Check sheet for the modelled part. Datum: model origin and axes. Units: mm. A direction names the side the tool comes from. Coordinates: 2 decimals unless noted, no trailing zeros. Loops run counter-clockwise (first coordinate to the right, second up) from the corner with the lowest first, then second, coordinate; pieces in that order, holes last.
from build123d import *

# Parameters (mm, degrees)
EXTRUDE_1_DEPTH     = 10
SKETCH_2_R          = 2
CUT_EXTRUDE_1_DEPTH = 13.051970793


with BuildPart() as part:
    # 草图1 → 凸台-拉伸1 (new body)
    with BuildSketch(Plane(origin=(0, 0, 0), x_dir=(1, 0, 0), z_dir=(0, 1, 0))):
        Polygon((-3.5, 0), (3.5, 0), (5, 1.5), (5, 3), (3, 3), (3, 4.5), (-3, 4.5), (-3, 3), (-5, 3), (-5, 1.5), align=None)
    extrude(amount=EXTRUDE_1_DEPTH)

    # 草图2 → 切除-拉伸1 (cut, through all)
    with BuildSketch(Plane.XY):
        with Locations((0, 5)):
            Circle(SKETCH_2_R)
    extrude(amount=-CUT_EXTRUDE_1_DEPTH, mode=Mode.SUBTRACT)


solid = part.part
(1) Section check A-A, the plane x = 0. Enter the section's corners in (y, z).
(2) Section check C-C, the plane y = 0.5. Enter the section's corners in (x, z), plus the area to 4 significant figures.
(3) Set-up check for faces 1 (the face through (3, 5, -4)), 2 (the face through (-5, 5, -2)), 3 (the face through (-3, 5, -4)): record each of +Z, -Z, +X, -X, +Y, -Y from which the full face is reachable in a straight line by a thin tool's end or side.
(4) Scan lines: line 1 along Y through (x, z) = (0, -0.2); line 2 along X through (y, z) = (0.5, -4); line 3 along X through (y, z) = (4.5, -2.95). Record each from-to range of solid material in increasing order.
(5) Section check D-D, the plane y = 5. Enter the section's corners in (x, z).
(6) Gauge pin test, flat ends, axial feed: P1, Ø1, axis at x = 4, y = 6, coming from the -Z side; P2, Ø2.5, axis at x = 0, y = 5, coming from the -Z side; P3, Ø1.6, axis at y = 6, z = -4, coming from the -X side; P4, Ø0.8, axis at y = 3, z = -3.5, coming from the +X side. Record the tip position at first contact, or that the pin passes through.
(7) Section check B-B, the plane z = -0.6. Enter the section's corners in (x, y).
(8) Draft check along Y on faces 4 (the face through (4.2, 4.9, -0.7)), 5 (the face through (0, 0, -2)), 6 (the face through (0, 7, -2)). Enter one of: pulls with the +Y half, pulls with the -Y half, needs draft (parallel to the pull), parting line crosses it, or undercut.
Determined:
1. outline: (0, -4.5) - (3, -4.5) - (3, 0) - (0, 0) - close; (7, -4.5) - (10, -4.5) - (10, 0) - (7, 0) - close
2. outline: (-5, -3) - (-3, -3) - (-3, -4.5) - (3, -4.5) - (3, -3) - (5, -3) - (5, -1.5) - (3.5, 0) - (-3.5, 0) - (-5, -1.5) - close
2. area: 36.75 mm2
3. face 1: -Z, +X, +Y, -Y
3. face 2: +Z, -Z, -X, +Y, -Y
3. face 3: -Z, -X, +Y, -Y
4. line 1: y = 0 to 3, 7 to 10
4. line 2: x = -3 to 3
4. line 3: x = -5 to -1.94, 1.94 to 5
5. outline: (-5, -3) - (-3, -3) - (-3, -4.5) - (-2, -4.5) - (-2, 0) - (-3.5, 0) - (-5, -1.5) - close; (2, -4.5) - (3, -4.5) - (3, -3) - (5, -3) - (5, -1.5) - (3.5, 0) - (2, 0) - close
6. P1: stops at z = -3
6. P2: passes through
6. P3: stops at x = -3
6. P4: stops at x = 3
7. outline: (-4.1, 0) - (4.1, 0) - (4.1, 10) - (-4.1, 10) - close; hole circle Ø4 at (0, 5)
8. face 4: needs draft
8. face 5: pulls with the -Y half
8. face 6: undercut
